from build123d import *

# Parameters (mm, degrees)
SKETCH1_W           = 32.95
SKETCH1_H           = 24
BOSS_EXTRUDE1_DEPTH = 1.45
SKETCH3_R           = 4
CUT_EXTRUDE1_DEPTH  = 41.789765873
SKETCH4_R           = 1
CUT_EXTRUDE2_DEPTH  = 41.789765873
CIRPATTERN1_COUNT   = 8
SKETCH6_R           = 1.25
CUT_EXTRUDE3_DEPTH  = 1.45
SKETCH7_R           = 1.25
CUT_EXTRUDE4_DEPTH  = 1.45
CIRPATTERN2_COUNT   = 4
CIRPATTERN3_COUNT   = 8
SKETCH8_W           = 1.45
SKETCH8_H           = 27.5
BOSS_EXTRUDE2_DEPTH = 7.15
CUT_EXTRUDE5_REACH  = 45.771
SKETCH9_W           = 2.15
SKETCH9_H           = 3.5
BOSS_EXTRUDE3_DEPTH = 1.45
FILLET1_R           = 1.5
FILLET2_R           = 1.5
SKETCH12_R          = 1.25
CUT_EXTRUDE6_DEPTH  = 1.5
SKETCH13_R          = 1.25
CUT_EXTRUDE7_DEPTH  = 1.5
SKETCH14_R          = 1.25
CUT_EXTRUDE8_DEPTH  = 1.5
SKETCH15_R          = 1.25
CUT_EXTRUDE9_DEPTH  = 1.5
BOSS_EXTRUDE5_DEPTH = 1.45
FILLET3_R           = 1.5
FILLET4_R           = 1.5


with BuildPart() as part:
    # Sketch1 → Boss-Extrude1 (new body)
    with BuildSketch(Plane.XY):
        with Locations((16.475, 12)):
            Rectangle(SKETCH1_W, SKETCH1_H)
    extrude(amount=BOSS_EXTRUDE1_DEPTH)

    # Sketch3 → Cut-Extrude1 (cut, through all)
    with BuildSketch(Plane.XY.offset(1.45)):
        with Locations((16.475, 12)):
            Circle(SKETCH3_R)
    extrude(amount=-CUT_EXTRUDE1_DEPTH, mode=Mode.SUBTRACT)

    # Sketch4 → Cut-Extrude2 (cut, through all)
    with BuildSketch(Plane.XY.offset(1.45)):
        with Locations((16.475, 20)):
            Circle(SKETCH4_R)
    cut_extrude2 = extrude(amount=-CUT_EXTRUDE2_DEPTH, mode=Mode.SUBTRACT)

    # CirPattern1: Cut-Extrude2 ×8 about axis
    cirpattern1_axis = Axis((16.475, 12, 0), (0, 0, 1))
    for i in range(1, CIRPATTERN1_COUNT):
        add(cut_extrude2.rotate(cirpattern1_axis, i * 360 / CIRPATTERN1_COUNT), mode=Mode.SUBTRACT)

    # Sketch6 → Cut-Extrude3 (cut)
    with BuildSketch(Plane.XY.offset(1.45)):
        with Locations((24.475, 15.312868697)):
            Circle(SKETCH6_R)
    cut_extrude3 = extrude(amount=-CUT_EXTRUDE3_DEPTH, mode=Mode.SUBTRACT)

    # Sketch7 → Cut-Extrude4 (cut)
    with BuildSketch(Plane.XY.offset(1.45)):
        with Locations((24.475, 20)):
            Circle(SKETCH7_R)
    cut_extrude4 = extrude(amount=-CUT_EXTRUDE4_DEPTH, mode=Mode.SUBTRACT)

    # CirPattern2: Cut-Extrude4 ×4 about axis
    cirpattern2_axis = Axis((16.475, 12, 0), (0, 0, 1))
    for i in range(1, CIRPATTERN2_COUNT):
        add(cut_extrude4.rotate(cirpattern2_axis, i * 360 / CIRPATTERN2_COUNT), mode=Mode.SUBTRACT)

    # CirPattern3: Cut-Extrude3 ×8 about axis
    cirpattern3_axis = Axis((16.475, 12, 0), (0, 0, 1))
    for i in range(1, CIRPATTERN3_COUNT):
        add(cut_extrude3.rotate(cirpattern3_axis, i * 360 / CIRPATTERN3_COUNT), mode=Mode.SUBTRACT)

    # Sketch8 → Boss-Extrude2 (add)
    with BuildSketch(Plane.XY.offset(1.45)):
        with Locations((0.725, 13.75)):
            Rectangle(SKETCH8_W, SKETCH8_H)
    boss_extrude2 = extrude(amount=BOSS_EXTRUDE2_DEPTH)

    # Sketch9 → Cut-Extrude5 (cut, up to next)
    with BuildSketch(Plane.ZY, mode=Mode.PRIVATE) as cut_extrude5_sk1:
        with Locations((2.525, 25.75)):
            Rectangle(SKETCH9_W, SKETCH9_H)
    cut_extrude5_tool1 = extrude(cut_extrude5_sk1.sketch, amount=-CUT_EXTRUDE5_REACH, mode=Mode.PRIVATE) & part.part
    cut_extrude5 = cut_extrude5_tool1.solids().sort_by_distance((0, 25.75, 2.525))[0]
    add(cut_extrude5, mode=Mode.SUBTRACT)

    # Sketch11 → Boss-Extrude3 (add)
    with BuildSketch(Plane(origin=(1.45, 0, 0), x_dir=(0, 0, -1), z_dir=(1, 0, 0))):
        Polygon((-3.6, 27.5), (-1.45, 24), (-3.6, 24), align=None)
    extrude(amount=-BOSS_EXTRUDE3_DEPTH)

    # Fillet1
    fillet1_edges = [part.edges().sort_by_distance(p)[0] for p in [
        (0.725, 0, 8.6),
        (0.725, 27.5, 8.6),
        (0.725, 27.5, 3.6),
        (0.725, 24, 1.45),
    ]]
    fillet(fillet1_edges, radius=FILLET1_R)

    # Fillet2
    fillet2_edges = [part.edges().sort_by_distance(p)[0] for p in [
        (0, 12, 0),
    ]]
    fillet(fillet2_edges, radius=FILLET2_R)

    # Sketch12 → Cut-Extrude6 (cut)
    with BuildSketch(Plane.ZY):
        with Locations((5.8, 4.2)):
            Circle(SKETCH12_R)
    cut_extrude6 = extrude(amount=-CUT_EXTRUDE6_DEPTH, mode=Mode.SUBTRACT)

    # Sketch13 → Cut-Extrude7 (cut)
    with BuildSketch(Plane.ZY):
        with Locations((5.8, 21.2)):
            Circle(SKETCH13_R)
    cut_extrude7 = extrude(amount=-CUT_EXTRUDE7_DEPTH, mode=Mode.SUBTRACT)

    # Sketch14 → Cut-Extrude8 (cut)
    with BuildSketch(Plane.ZY):
        with Locations((5.8, 25.1)):
            Circle(SKETCH14_R)
    cut_extrude8 = extrude(amount=-CUT_EXTRUDE8_DEPTH, mode=Mode.SUBTRACT)

    # Sketch15 → Cut-Extrude9 (cut)
    with BuildSketch(Plane.ZY):
        with Locations((5.8, 8.1)):
            Circle(SKETCH15_R)
    cut_extrude9 = extrude(amount=-CUT_EXTRUDE9_DEPTH, mode=Mode.SUBTRACT)

    # Mirror3: Boss-Extrude2 across plane
    add(boss_extrude2.mirror(Plane(origin=(16.475, 0, 0), x_dir=(0, 0, 1), z_dir=(1, 0, 0))))

    # Mirror5: Cut-Extrude5 across plane
    add(cut_extrude5.mirror(Plane(origin=(16.475, 0, 0), x_dir=(0, 0, 1), z_dir=(1, 0, 0))), mode=Mode.SUBTRACT)

    # Sketch17 → Boss-Extrude5 (add)
    with BuildSketch(Plane.ZY.offset(-31.5)):
        Polygon((1.45, 24), (3.6, 27.5), (3.6, 24), align=None)
    extrude(amount=-BOSS_EXTRUDE5_DEPTH)

    # Mirror8: Cut-Extrude6, Cut-Extrude7, Cut-Extrude8, Cut-Extrude9 across plane
    add(cut_extrude6.mirror(Plane(origin=(16.475, 0, 0), x_dir=(0, 0, 1), z_dir=(1, 0, 0))), mode=Mode.SUBTRACT)
    add(cut_extrude7.mirror(Plane(origin=(16.475, 0, 0), x_dir=(0, 0, 1), z_dir=(1, 0, 0))), mode=Mode.SUBTRACT)
    add(cut_extrude8.mirror(Plane(origin=(16.475, 0, 0), x_dir=(0, 0, 1), z_dir=(1, 0, 0))), mode=Mode.SUBTRACT)
    add(cut_extrude9.mirror(Plane(origin=(16.475, 0, 0), x_dir=(0, 0, 1), z_dir=(1, 0, 0))), mode=Mode.SUBTRACT)

    # Fillet3
    fillet3_edges = [part.edges().sort_by_distance(p)[0] for p in [
        (32.225, 27.5, 8.6),
        (32.225, 0, 8.6),
        (32.225, 27.5, 3.6),
        (32.225, 24, 1.45),
    ]]
    fillet(fillet3_edges, radius=FILLET3_R)

    # Fillet4
    fillet4_edges = [part.edges().sort_by_distance(p)[0] for p in [
        (32.95, 12, 0),
    ]]
    fillet(fillet4_edges, radius=FILLET4_R)


solid = part.part
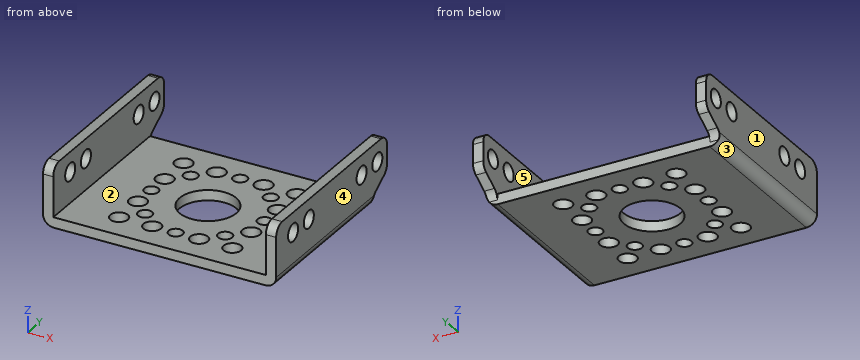
CAD build for the part. Positions are in the model's coordinates, mm. Face numbers are marked on the shaded views. A direction names the side the tool comes from. Coordinates: 2 decimals unless noted, no trailing zeros. Write each loop counter-clockwise with the first axis right and the second up, starting at its lowest first coordinate (ties: lowest second). Pieces come first, ordered by that corner, then holes. Notation, with made-up numbers: M 53.5,40 L 89.5,40 A16 ccw 89.5,44 Z; hole C 15,-16 d4. An arc over 180 degrees is marked long. Return JSON: item names as keys, results as strings.
Item 1: Slice it at C-C, the plane y = 19.5. State how many separate pieces and enclosed holes the cut face has, and give its area (3 significant figures).
Findings below:
{"separate pieces": "6", "enclosed holes": "0", "area": "51.7 mm2"}
Item 2: Drop flat-ended pins along their axis: pin 1 Ø3 at (x, y) = (22.13, 17.66) entering from +Z; pin 2 Ø1.2 at (x, z) = (9.5, 0.5) entering from +Y. Give the stop position or say it passes through.
Findings below:
{"pin 1": "stops at z = 1.45", "pin 2": "stops at y = 24"}
Item 3: Which spindle directions (+Z, -Z, +X, -X, +Y, -Y) get a long thin tool onto all of the face, cutting with end or side? Do the marked faces 1 and 2. Say none if no direction does.
Findings below:
{"face 1": "+Z, -Z, -X, +Y, -Y", "face 2": "+Z, +Y, -Y"}
Item 4: Slice it at A-A, the plane y = 25.1. Write the cut outline in (x, z), and give its area (3 significant figures).
Findings below:
{"outline": "M 0,2.13 L 1.45,2.13 L 1.45,4.55 L 0,4.55 Z; M 0,7.05 L 1.45,7.05 L 1.45,8.6 L 0,8.6 Z; M 31.5,2.13 L 32.95,2.13 L 32.95,4.55 L 31.5,4.55 Z; M 31.5,7.05 L 32.95,7.05 L 32.95,8.6 L 31.5,8.6 Z", "area": "11.5 mm2"}
Item 5: Probe line 1 (Y direction, x = 32.1, z = 5.8); line 2 (X direction, y = 4, z = 2.25); line 3 (Y direction, x = 19, z = 1). List the from-to ranges inside material, lowest first. Write a range as from..to.
Findings below:
{"line 1": "y = 0..2.95, 5.45..6.85, 9.35..19.95, 22.45..23.85, 26.35..27.5", "line 2": "x = 0..1.45, 31.5..32.95", "line 3": "y = 0..3.03, 4.97..8.9, 15.1..19.03, 20.97..24"}
Item 6: Slice it at D-D, the plane z = 4. Write the cut outline in (x, y).
Findings below:
{"outline": "M 0,0 L 1.45,0 L 1.45,27.43 L 0,27.43 Z; M 31.5,0 L 32.95,0 L 32.95,27.43 L 31.5,27.43 Z"}
Item 7: Slice it at B-B, the plane x = 9. Write the cut outline in (y, z).
Findings below:
{"outline": "M 0,0 L 2.87,0 L 2.87,1.45 L 0,1.45 Z; M 5.13,0 L 7.55,0 L 7.55,1.45 L 5.13,1.45 Z; M 9.82,0 L 11.15,0 L 11.15,1.45 L 9.82,1.45 Z; M 12.85,0 L 14.18,0 L 14.18,1.45 L 12.85,1.45 Z; M 16.45,0 L 18.87,0 L 18.87,1.45 L 16.45,1.45 Z; M 21.13,0 L 24,0 L 24,1.45 L 21.13,1.45 Z"}
Item 8: Two-plate mould, pull along X, no slides. Class the marked faces 3, 4 and 5: +X half, -X half, draft (parallel to the pull), parting line (faces both ways), or undercut.
Findings below:
{"face 3": "-X half", "face 4": "+X half", "face 5": "undercut"}
